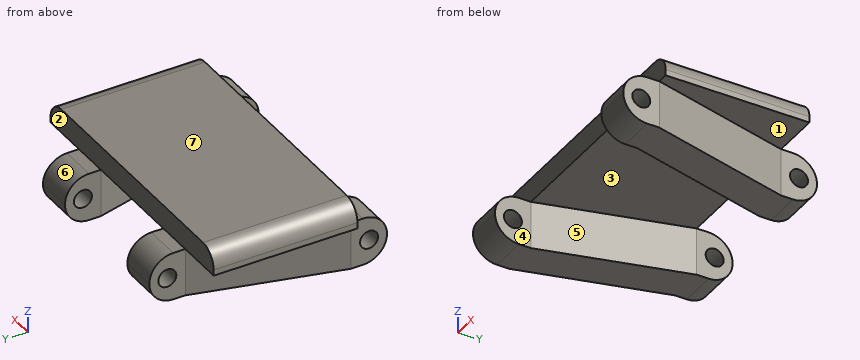
```python
from build123d import *

# Parameters (mm, degrees)
SKETCH2_W                      = 23
SKETCH2_H                      = 12
BOSS_EXTRUDE2_DEPTH            = 2
FILLET3_R                      = 1.5
BOSS_EXTRUDE4_DEPTH            = 4
FILLET4_R                      = 2
F_1_5MM_DOWEL_HOLE1_AT_2_COUNT = 2
F_1_5MM_DOWEL_HOLE1_AT_2_PITCH = 15
F_1_5MM_DOWEL_HOLE2_D          = 1.5
F_1_5MM_DOWEL_HOLE2_DEPTH      = 29999.549354536
F_1_5MM_DOWEL_HOLE2_TIP        = 0.450645464


with BuildPart() as part:
    # Sketch2 → Boss-Extrude2 (new body)
    with BuildSketch(Plane.XY):
        Rectangle(SKETCH2_W, SKETCH2_H)
    extrude(amount=BOSS_EXTRUDE2_DEPTH)

    # Fillet3
    fillet3_edges = [part.edges().sort_by_distance(p)[0] for p in [
        (-11.5, 0, 2),
        (11.5, 0, 2),
    ]]
    fillet(fillet3_edges, radius=FILLET3_R)

    # Sketch3 → Boss-Extrude4 (add)
    with BuildSketch(Plane(origin=(0, 0, 0), x_dir=(-1, 0, 0), z_dir=(0, 0, -1))):
        Polygon((-10.602604408, -6), (-7.5, 6), (-7.5, 9), (-4.401349547, 9), (-4.401349547, 6), (-7.503953954, -6), (-7.503953954, -9), (-10.602604408, -9), align=None)
        Polygon((7.503953954, -6), (4.401349547, 6), (4.401349547, 9), (7.5, 9), (7.5, 6), (10.602604408, -6), (10.602604408, -9), (7.503953954, -9), align=None)
    extrude(amount=BOSS_EXTRUDE4_DEPTH)

    # Fillet4
    fillet4_edges = [part.edges().sort_by_distance(p)[0] for p in [
        (-9.053279181, -9, 0),
        (-9.053279181, -9, -4),
        (9.053279181, -9, 0),
        (9.053279181, -9, -4),
        (5.950674773, 9, 0),
        (5.950674773, 9, -4),
        (-5.950674773, 9, 0),
        (-5.950674773, 9, -4),
    ]]
    fillet(fillet4_edges, radius=FILLET4_R - 0.0001)  # a hair under: the kernel refuses the full size

    # Sketch9 → Ø1.5mm Dowel Hole1 (revolve, cut)
    with BuildSketch(Plane(origin=(7.5, 7.5, -2), x_dir=(0, 0, -1), z_dir=(0, 1, 0))):
        Polygon((0, 0), (0, 30000), (0.75, 29999.549354536), (0.75, 0), align=None)
    f_1_5mm_dowel_hole1 = revolve(axis=Axis((13.85, 7.5, -2), (-1, 0, 0)), mode=Mode.SUBTRACT)

    # Ø1.5mm Dowel Hole1 at 2: Ø1.5mm Dowel Hole1 ×2
    with Locations(*[(0, -i * F_1_5MM_DOWEL_HOLE1_AT_2_PITCH, 0) for i in range(1, F_1_5MM_DOWEL_HOLE1_AT_2_COUNT)]):
        add(f_1_5mm_dowel_hole1, mode=Mode.SUBTRACT)

    # Ø1.5mm Dowel Hole2
    with Locations(Plane(origin=(7.5, -7.5, -2), x_dir=(0, 0, -1), z_dir=(-1, 0, 0))):
        with Locations((0, 0)):
            Hole(F_1_5MM_DOWEL_HOLE2_D / 2, depth=F_1_5MM_DOWEL_HOLE2_DEPTH)
            with Locations((0, 0, -(F_1_5MM_DOWEL_HOLE2_DEPTH + F_1_5MM_DOWEL_HOLE2_TIP / 2))):  # 118° drill point
                Cone(0, F_1_5MM_DOWEL_HOLE2_D / 2, F_1_5MM_DOWEL_HOLE2_TIP, mode=Mode.SUBTRACT)


solid = part.part
```
Could you check a few things on this model? Use its own coordinates, in mm. Face numbers are marked on the shaded views. A direction names the side the tool comes from. Give positions to 0.01 mm unless a question says otherwise; leave off trailing zeros. Loops run counter-clockwise (first coordinate to the right, second up) from the corner with the lowest first, then second, coordinate; pieces in that order, holes last. Notation, with made-up numbers: (64.25, 10.25) - (68.25, 10.25) arc R29 ccw to (68.25, 46.25) - close; hole circle Ø7 at (-13.5, 61.5). An arc over 180 degrees is marked (long way). Answer in a Markdown table with one row per item. Add a question column.
Q1. If we section it at C-C (y = -7.5): List the corners of the cut face in (x, z) for me.
Q2. If we section it at B-B (z = -2.25): State how many separate pieces and enclosed holes the cut face has, plus the area to 3 significant figures.
Q3. Which directions (+Z, -Z, +X, -X, +Y, -Y) give clear straight access to the entire face, cutting with the end or side of a thin tool? Please do the marked faces 1, 2, 3 and 4.
Q4. For pin 1 (0.9 mm diameter, centred on y = -8, z = -2, fed in from +X); pin 2 (2.5 mm diameter, centred on y = 7.5, z = -1.5, fed in from -X); pin 3 (1 mm diameter, centred on x = 3, z = 1, fed in from +Y), each with a flat end and sliding along its axis, tell me the tip position at first contact or that it passes through.
Q5. We'd pull the mould along Y, two halves only. Please class the marked faces 5, 6 and 7: +Y half, -Y half, draft (parallel to the pull), parting line (faces both ways), or undercut.
Q6. If we section it at D-D (y = 3): List the corners of the cut face in (x, z) for me, plus the area to 3 significant figures.
Q7. Please list where these lines run through material, in increasing order: L1, parallel to X at y = -7, z = -0.25; L2, parallel to Z at x = -1.5, y = 1; L3, parallel to Z at x = 6.6, y = 7.5. Write a range as from..to.
The answers:
| question | item | result |
|---|---|---|
| 1 | outline | (-10.6, -3.94) - (-7.5, -3.94) - (-7.5, -2.75) - (-10.6, -2.75) - close; (-10.6, -1.25) - (-7.5, -1.25) - (-7.5, -0.06) - (-10.6, -0.06) - close; (7.5, -3.94) - (10.6, -3.94) - (10.6, -2.75) - (7.5, -2.75) - close; (7.5, -1.25) - (10.6, -1.25) - (10.6, -0.06) - (7.5, -0.06) - close |
| 2 | separate pieces | 6 |
| 2 | enclosed holes | 0 |
| 2 | area | 93.8 mm^2 |
| 3 | face 1 | -Z, +X, +Y |
| 3 | face 2 | +Z, +X, -X, +Y |
| 3 | face 3 | -Z, -Y |
| 3 | face 4 | +Z, -Z, -Y |
| 4 | pin 1 | stops at x = 10.6 |
| 4 | pin 2 | stops at x = -7.5 |
| 4 | pin 3 | stops at y = 6 |
| 5 | face 5 | -Y half |
| 5 | face 6 | +Y half |
| 5 | face 7 | draft |
| 6 | outline | (-11.5, 0) - (-8.28, 0) - (-8.28, -4) - (-5.18, -4) - (-5.18, 0) - (5.18, 0) - (5.18, -4) - (8.28, -4) - (8.28, 0) - (11.5, 0) - (11.5, 0.5) arc R1.5 ccw to (10, 2) - (-10, 2) arc R1.5 ccw to (-11.5, 0.5) - close |
| 6 | area | 69.8 mm^2 |
| 7 | L1 | x = -10.6..-7.5, 7.5..10.6 |
| 7 | L2 | z = 0..2 |
| 7 | L3 | z = -3.94..-2.75, -1.25..-0.06 |
